Could you check a few things on this model? Use its own coordinates, in mm. A direction names the side the tool comes from. Give positions to 0.01 mm unless a question says otherwise; leave off trailing zeros. Order: outer loops, then holes, each group sorted by start corner. A loop starts at its lowest first (then second) coordinate and runs counter-clockwise, first axis right, second up.
from build123d import *

# Parameters (mm, degrees)
SKETCH2_OUTSIDE_W       = 99.054
SKETCH2_OUTSIDE_H       = 99.054
SKETCH2_OUTSIDE_R       = 20
CUT_EXTRUDE1_DEPTH      = 5
CUT_EXTRUDE2_DEPTH      = 98.002577285
CUT_EXTRUDE2_DEPTH_BACK = 7
SKETCH3_R               = 17.75
CUT_EXTRUDE3_DEPTH      = 40
SKETCH5_R               = 4
CUT_EXTRUDE4_DEPTH      = 10
SKETCH6_R               = 21
CUT_EXTRUDE6_DEPTH      = 76


with BuildPart() as part:
    # Sketch1 → Revolve1 (revolve)
    with BuildSketch(Plane.XY, mode=Mode.PRIVATE) as revolve1_sk:
        with BuildLine():
            Line((0, -83), (28, -83))
            Line((28, -83), (28, -71))
            Line((28, -71), (26.7, -68.5))
            ThreePointArc((26.7, -68.5), (28, -66.23203125), (27.35, -63.7))
            ThreePointArc((27.35, -63.7), (26.7, -61.3), (27.35, -58.9))
            ThreePointArc((27.35, -58.9), (28, -56.5), (27.35, -54.1))
            ThreePointArc((27.35, -54.1), (26.558436035, -51.7), (27.35, -49.3))
            ThreePointArc((27.35, -49.3), (28, -46.76796875), (26.7, -44.5))
            Line((26.7, -44.5), (28, -42))
            Line((28, -42), (28, -40))
            ThreePointArc((28, -40), (29.936654182, -29.319995318), (35.5, -20))
            Line((35.5, -20), (35.5, 0))
            Line((35.5, 0), (0, 0))
            Line((0, 0), (0, -83))
        make_face()
    revolve(revolve1_sk.sketch.rotate(Axis((0, 0, 0), (0, -1, 0)), 90), axis=Axis((0, 0, 0), (0, -1, 0)))

    # Sketch2 outside → Cut-Extrude1 (cut)
    with BuildSketch(Plane(origin=(0, 0, 0), x_dir=(1, 0, 0), z_dir=(0, 1, 0))):
        Rectangle(SKETCH2_OUTSIDE_W, SKETCH2_OUTSIDE_H)
        with Locations(Location((0, 0, 0), (0, 0, 270))):
            Circle(SKETCH2_OUTSIDE_R, mode=Mode.SUBTRACT)
    extrude(amount=-CUT_EXTRUDE1_DEPTH, mode=Mode.SUBTRACT)

    # Sketch3 → Cut-Extrude2 (cut, two sides: drawn at the far end of the back side and taken through both)
    with BuildSketch(Plane(origin=(0, 0, 0), x_dir=(1, 0, 0), z_dir=(0, 1, 0)).offset(-CUT_EXTRUDE2_DEPTH_BACK)):
        with Locations(Location((0, 0, 0), (0, 0, 90))):
            Circle(SKETCH3_R)
    extrude(amount=CUT_EXTRUDE2_DEPTH + CUT_EXTRUDE2_DEPTH_BACK, mode=Mode.SUBTRACT)

    # Sketch4 → Cut-Extrude3 (cut)
    with BuildSketch(Plane(origin=(0, -5, 0), x_dir=(1, 0, 0), z_dir=(0, 1, 0))):
        with BuildLine():
            Line((-11.5, 27.708302005), (-11.5, 36.893569163))
            ThreePointArc((-11.5, 36.893569163), (-38.452583445, 21.587967058), (-39.116292786, -9.400138727))
            Line((-39.116292786, -9.400138727), (-29.746093432, -3.894858859))
            ThreePointArc((-29.746093432, -3.894858859), (-25.980762114, 15), (-11.5, 27.708302005))
        make_face()
        with BuildLine():
            Line((11.5, 27.708302005), (11.5, 36.893569163))
            Line((11.5, 36.893569163), (28.492131838, 31.542661949))
            Line((28.492131838, 31.542661949), (37.637433316, 13.990056046))
            Line((37.637433316, 13.990056046), (44.445273929, 4.335643403))
            Line((44.445273929, 4.335643403), (37.637433316, -8.052167996))
            Line((37.637433316, -8.052167996), (34.836079144, -6.83356348))
            Line((34.836079144, -6.83356348), (29.746093432, -3.894858859))
            ThreePointArc((29.746093432, -3.894858859), (25.980762114, 15), (11.5, 27.708302005))
        make_face()
        with BuildLine():
            Line((-18.246093432, -23.813443146), (-23.336079144, -26.752147767))
            Line((-23.336079144, -26.752147767), (-24.985631262, -28.64317075))
            Line((-24.985631262, -28.64317075), (-15.892945892, -35.329052408))
            Line((-15.892945892, -35.329052408), (-5.348602182, -38.036383901))
            Line((-5.348602182, -38.036383901), (8.188055284, -38.036383901))
            Line((8.188055284, -38.036383901), (20.43638373, -32.98577886))
            Line((20.43638373, -32.98577886), (24.324755582, -27.697659259))
            Line((24.324755582, -27.697659259), (23.336079144, -26.752147767))
            Line((23.336079144, -26.752147767), (18.246093432, -23.813443146))
            ThreePointArc((18.246093432, -23.813443146), (0, -30), (-18.246093432, -23.813443146))
        make_face()
    extrude(amount=-CUT_EXTRUDE3_DEPTH, mode=Mode.SUBTRACT)

    # Sketch5 → Cut-Extrude4 (cut)
    with BuildSketch(Plane(origin=(0, -5, 0), x_dir=(1, 0, 0), z_dir=(0, 1, 0))):
        with Locations(Location((0, 28, 0), (0, 0, 270))):
            Circle(SKETCH5_R)
        with Locations(Location((24.248711306, -14, 0), (0, 0, 270))):
            Circle(SKETCH5_R)
        with Locations(Location((-24.248711306, -14, 0), (0, 0, 270))):
            Circle(SKETCH5_R)
    extrude(amount=-CUT_EXTRUDE4_DEPTH, mode=Mode.SUBTRACT)

    # Sketch6 → Cut-Extrude6 (cut)
    with BuildSketch(Plane.XZ.offset(83)):
        with Locations(Location((0, 0, 0), (0, 0, 270))):
            Circle(SKETCH6_R)
    extrude(amount=-CUT_EXTRUDE6_DEPTH, mode=Mode.SUBTRACT)


solid = part.part
Item 1: Imagine slicing it at A-A on y = -77.5. List the corners of the cut face in (x, z) for me, then the cut area to 3 significant figures.
Findings:
outline: circle Ø56 at (0, 0); hole circle Ø42 at (0, 0)
area: 1,080 mm2
Item 2: For pin 1 (2 mm diameter, centred on y = -43.5, z = -22.5, fed in from -X); pin 2 (3 mm diameter, centred on y = -11.5, z = -31.5, fed in from -X); pin 3 (1.8 mm diameter, centred on y = -15, z = -31.5, fed in from +X), each with a flat end and sliding along its axis, tell me the tip position at first contact or that it passes through.
Findings:
pin 1: stops at x = -16.95
pin 2: stops at x = -11.5
pin 3: stops at x = 11.5
Item 3: For faces 4 (the cylindrical face through (15.747, -3.549, -8.191)), 5 (the cylindrical face through (24.84, -76.92, 12.92)), 6 (the flat face through (11.5, -14, -31)), 7 (the flat face through (20.827, -14.224, 25.303)), 8 (the flat face through (24, -15, 14)), which set-ups out of +Z, -Z, +X, -X, +Y, -Y let a thin tool reach every point of the face, with its end or its side?
Findings:
face 4: +Y, -Y
face 5: -Y
face 6: -Z, +X, +Y, -Y
face 7: +Z, +Y, -Y
face 8: +Y
Item 4: Please list where these lines run through material, in increasing order: line 1 along Z through (x, y) = (-3, -8); line 2 along X through (y, z) = (-7, -28); line 3 along Y through (x, z) = (15.5, -13).
Findings:
line 1: z = -35.37 to -30.65, -25.35 to -20.78, 20.78 to 29.85
line 2: x = -11.5 to -4, 4 to 11.5
line 3: y = -7 to -5
Item 5: We'd pull the mould along X, two halves only. Please class faces 1 (the conical face through (26.144, -44.344, -5.806)), 2 (the flat face through (0, -15, -28)), 3 (the flat face through (-32.322, -14.224, 5.408)): +X half, -X half, draft (parallel to the pull), parting line (faces both ways), or undercut.
Findings:
face 1: parting line
face 2: undercut
face 3: -X half
Item 6: Imagine slicing it at B-B on y = -38.5. List the corners of the cut face in (x, z) for me.
Findings:
outline: circle Ø56.07 at (0, 0); hole circle Ø42 at (0, 0)
